Part print with two shaded views. Sizes in mm from the minimum x, y, z corner. A direction names the side the tool comes from. Give positions to 0.01 mm unless a question says otherwise; leave off trailing zeros. Order: outer loops, then holes, each group sorted by start corner. A loop starts at its lowest first (then second) coordinate and runs counter-clockwise, first axis right, second up.
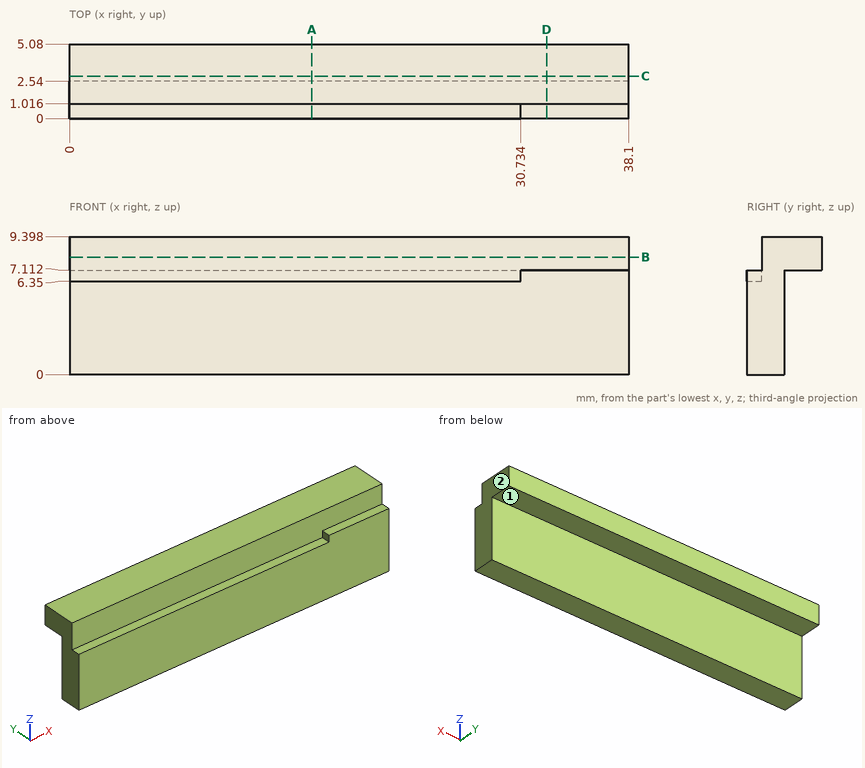
1. 3-axis set-ups, long thin cutter, end or side, ignore diameter. For the marked faces 1 and 2: which of +Z, -Z, +X, -X, +Y, -Y reach the whole face in a straight line?
2. Wall check: line 1 (Y direction, x = 13, z = 0.5); line 2 (Y direction, x = 5, z = 7); line 3 (Z direction, x = 21, y = 0.4). Give the ranges that are in metal, low to high.
3. Saw through at B-B on z = 8. Give the cut face in (x, y).
4. Saw through at A-A on x = 16.5. Give the cut face in (y, z), plus the area to 3 significant figures.
5. Saw through at D-D on x = 32.5. Give the cut face in (y, z), plus the area to 3 significant figures.
6. Pin check, flat tips, straight feed: P1, Ø1.3, axis at x = 14.5, y = 4, coming from the -Z side; P2, Ø0.5, axis at x = 33, y = 0.5, coming from the +Z side; P3, Ø1, axis at x = 27.5, z = 6, coming from the +Y side. Stop position of each tip, or through.
7. Saw through at C-C on y = 2.9. Give the cut face in (x, z), plus the area to 3 significant figures.
Reported:
1. face 1: -Z, +X, -X, +Y
1. face 2: +Z, -Z, +X, +Y, -Y
2. line 1: y = 0 to 2.54
2. line 2: y = 1.02 to 2.54
2. line 3: z = 0 to 6.35
3. outline: (0, 1.02) - (38.1, 1.02) - (38.1, 5.08) - (0, 5.08) - close
4. outline: (0, 0) - (2.54, 0) - (2.54, 7.11) - (5.08, 7.11) - (5.08, 9.4) - (1.02, 9.4) - (1.02, 6.35) - (0, 6.35) - close
4. area: 26.6 mm2
5. outline: (0, 0) - (2.54, 0) - (2.54, 7.11) - (5.08, 7.11) - (5.08, 9.4) - (1.02, 9.4) - (1.02, 7.11) - (0, 7.11) - close
5. area: 27.4 mm2
6. P1: stops at z = 7.11
6. P2: stops at z = 7.11
6. P3: stops at y = 2.54
7. outline: (0, 7.11) - (38.1, 7.11) - (38.1, 9.4) - (0, 9.4) - close
7. area: 87.1 mm2
